CAD build for the part. Positions are in the model's coordinates, mm. A direction names the side the tool comes from. Give positions to 0.01 mm unless a question says otherwise; leave off trailing zeros. Loops run counter-clockwise (first coordinate to the right, second up) from the corner with the lowest first, then second, coordinate; pieces in that order, holes last.
Item 1: Which spindle directions (+Z, -Z, +X, -X, +Y, -Y) get a long thin tool onto all of the face, cutting with end or side? Do faces 1 (the flat face through (-18.25, 91, -7)), 2 (the flat face through (0, 38.624, 0)), 3 (the flat face through (-26, 51, -14.811)). Say none if no direction does.
Item 2: Mould opens along X. For faces 4 (the flat face through (-23, 83.033, -12)), 5 (the flat face through (0, 72.984, 0)), 6 (the flat face through (0, 86.208, -1)), 7 (the flat face through (30.95, 49, -7)) say: released by +X, released by -X, zero draft, split by the parting line, or undercut.
Item 3: Saw through at B-B on z = 0.75. Give the cut face in (x, y).
Item 4: Saw through at C-C on x = 1. Give the cut face in (y, z), plus the area to 3 significant figures.
Item 5: Saw through at D-D on z = -7.75. Give the cut face in (x, y).
Item 6: Drop flat-ended pins along their axis: P1, Ø1, axis at x = 29, y = 12, coming from the -Z side; P2, Ø10, axis at x = 17, y = 15, coming from the -Z side; P3, Ø5, axis at x = -25, z = -10.5, coming from the -Y side; P4, Ø5.5, axis at x = 13, z = -0.5, coming from the -Y side. Give the stop position or say it passes through.
Item 7: Saw through at A-A on y = 91.5. Give the cut face in (x, z).
Item 8: Probe probe 1 along Y at (x, z) = (-16, -2.5); probe 2 along X at (y, z) = (30, -14); probe 3 along Z at (x, y) = (27, 78). List the from-to ranges inside material, lowest first.
from build123d import *

# Parameters (mm, degrees)
BOSS_EXTRUDE1_DEPTH = 83.0326
SKETCH6_W           = 61.8998
SKETCH6_H           = 21.463
BOSS_EXTRUDE3_DEPTH = 3.175
SKETCH7_W           = 16.5354
SKETCH7_H           = 9.525
CUT_EXTRUDE2_DEPTH  = 91.420129415
SKETCH8_W           = 5.08
SKETCH8_H           = 25.4
CUT_EXTRUDE3_DEPTH  = 108.64212172
SKETCH15_W          = 61.8998
SKETCH15_H          = 20.63242
CUT_EXTRUDE4_DEPTH  = 3.175
SKETCH16_W          = 36.4998
SKETCH16_H          = 12.7
CUT_EXTRUDE5_DEPTH  = 3.175
SKETCH17_W          = 12.7
SKETCH17_H          = 21.463
BOSS_EXTRUDE4_DEPTH = 12.7


with BuildPart() as part:
    # Sketch1 → Boss-Extrude1 (new body)
    with BuildSketch(Plane(origin=(0, 0, 0), x_dir=(1, 0, 0), z_dir=(0, 1, 0))):
        Polygon((-30.9499, -3.477149156), (30.9499, -3.477149156), (30.9499, 17.985850844), (24.0411, 17.985850844), (24.0411, 14.810850844), (27.7749, 14.810850844), (27.7749, 5.285850844), (-27.7749, 5.285850844), (-27.7749, 14.810850844), (-24.0411, 14.810850844), (-24.0411, 17.985850844), (-30.9499, 17.985850844), align=None)
    extrude(amount=BOSS_EXTRUDE1_DEPTH)

    # Sketch6 → Boss-Extrude3 (add)
    with BuildSketch(Plane(origin=(0, 83.0326, 0), x_dir=(1, 0, 0), z_dir=(0, 1, 0))):
        with Locations((0, 7.254350844)):
            Rectangle(SKETCH6_W, SKETCH6_H)
    extrude(amount=BOSS_EXTRUDE3_DEPTH)

    # Sketch7 → Cut-Extrude2 (cut, through all)
    with BuildSketch(Plane.XZ.offset(-83.0326)):
        with Locations((0, -10.048350844)):
            Rectangle(SKETCH7_W, SKETCH7_H)
    extrude(amount=-CUT_EXTRUDE2_DEPTH, mode=Mode.SUBTRACT)

    # Sketch8 → Cut-Extrude3 (cut, through all)
    with BuildSketch(Plane.ZY.offset(30.9499)):
        with Locations((-0.274453158, 60.28364576)):
            Rectangle(SKETCH8_W, SKETCH8_H)
        with Locations((-0.274453158, 25.92395424)):
            Rectangle(SKETCH8_W, SKETCH8_H)
    extrude(amount=-CUT_EXTRUDE3_DEPTH, mode=Mode.SUBTRACT)

    # Sketch15 → Cut-Extrude4 (cut)
    with BuildSketch(Plane(origin=(0, 0, -17.985850844), x_dir=(-1, 0, 0), z_dir=(0, 0, -1))):
        with Locations((0, 10.31621)):
            Rectangle(SKETCH15_W, SKETCH15_H)
    extrude(amount=-CUT_EXTRUDE4_DEPTH, mode=Mode.SUBTRACT)

    # Sketch16 → Cut-Extrude5 (cut)
    with BuildSketch(Plane(origin=(0, 86.2076, 0), x_dir=(1, 0, 0), z_dir=(0, 1, 0))):
        with Locations((0, 11.635850844)):
            Rectangle(SKETCH16_W, SKETCH16_H)
    extrude(amount=-CUT_EXTRUDE5_DEPTH, mode=Mode.SUBTRACT)

    # Sketch17 → Boss-Extrude4 (add)
    with BuildSketch(Plane(origin=(0, 86.2076, 0), x_dir=(1, 0, 0), z_dir=(0, 1, 0))):
        with Locations((-24.5999, 7.254350844)):
            Rectangle(SKETCH17_W, SKETCH17_H)
        with Locations((24.5999, 7.254350844)):
            Rectangle(SKETCH17_W, SKETCH17_H)
    extrude(amount=BOSS_EXTRUDE4_DEPTH)


solid = part.part
Results below:
1. face 1: -Z, +Y
1. face 2: +X, -X
1. face 3: -Y
2. face 4: undercut
2. face 5: zero draft
2. face 6: undercut
2. face 7: released by +X
3. outline: (-30.95, 0) - (30.95, 0) - (30.95, 13.22) - (-30.95, 13.22) - close; (-30.95, 38.62) - (30.95, 38.62) - (30.95, 47.58) - (-30.95, 47.58) - close; (-30.95, 72.98) - (30.95, 72.98) - (30.95, 98.91) - (18.25, 98.91) - (18.25, 86.21) - (-18.25, 86.21) - (-18.25, 98.91) - (-30.95, 98.91) - close
4. outline: (0, -5.29) - (86.21, -5.29) - (86.21, 3.48) - (0, 3.48) - close; hole (13.22, -2.81) - (38.62, -2.81) - (38.62, 2.27) - (13.22, 2.27) - close; hole (47.58, -2.81) - (72.98, -2.81) - (72.98, 2.27) - (47.58, 2.27) - close
4. area: 497 mm2
5. outline: (-30.95, 0) - (-27.77, 0) - (-27.77, 83.03) - (-18.25, 83.03) - (-18.25, 98.91) - (-30.95, 98.91) - close; (18.25, 83.03) - (27.77, 83.03) - (27.77, 0) - (30.95, 0) - (30.95, 98.91) - (18.25, 98.91) - close
6. P1: stops at z = -14.81
6. P2: stops at z = -5.29
6. P3: stops at y = 83.03
6. P4: stops at y = 0
7. outline: (-30.95, -17.99) - (-18.25, -17.99) - (-18.25, 3.48) - (-30.95, 3.48) - close; (18.25, -17.99) - (30.95, -17.99) - (30.95, 3.48) - (18.25, 3.48) - close
8. probe 1: y = 0 to 13.22, 38.62 to 47.58, 72.98 to 86.21
8. probe 2: x = -30.95 to -27.77, 27.77 to 30.95
8. probe 3: z = -17.99 to -14.81, -5.29 to 3.48
